```python
from build123d import *

# Parameters (mm, degrees)
SKETCH1_W           = 86
SKETCH1_H           = 40
BOSS_EXTRUDE1_DEPTH = 1.3
SKETCH2_W           = 1.4
SKETCH2_H           = 22
BOSS_EXTRUDE2_DEPTH = 1.3
CUT_EXTRUDE1_DEPTH  = 49.713961038
BOSS_EXTRUDE3_DEPTH = 1.3


with BuildPart() as part:
    # Sketch1 → Boss-Extrude1 (new body)
    with BuildSketch(Plane(origin=(0, 0, 0), x_dir=(1, 0, 0), z_dir=(0, 1, 0))):
        Rectangle(SKETCH1_W, SKETCH1_H)
    extrude(amount=BOSS_EXTRUDE1_DEPTH)

    # Sketch2 → Boss-Extrude2 (add)
    with BuildSketch(Plane(origin=(0, 1.3, 0), x_dir=(1, 0, 0), z_dir=(0, 1, 0))):
        with Locations((-43.7, -3)):
            Rectangle(SKETCH2_W, SKETCH2_H)
        with Locations((43.7, -3)):
            Rectangle(SKETCH2_W, SKETCH2_H)
    extrude(amount=-BOSS_EXTRUDE2_DEPTH)

    # Sketch3 → Cut-Extrude1 (cut, through all)
    with BuildSketch(Plane(origin=(0, 1.3, 0), x_dir=(1, 0, 0), z_dir=(0, 1, 0))):
        Polygon((29, 20), (-29, 20), (-11, -18), (11, -18), align=None)
    extrude(amount=-CUT_EXTRUDE1_DEPTH, mode=Mode.SUBTRACT)

    # Sketch4 → Boss-Extrude3 (add)
    with BuildSketch(Plane(origin=(0, 0, 0), x_dir=(1, 0, 0), z_dir=(0, 1, 0))):
        Polygon((-28, -20), (-18.75, -39.527777778), (18.75, -39.527777778), (28, -20), align=None)
    extrude(amount=BOSS_EXTRUDE3_DEPTH)


solid = part.part
```
Geometry: final body of the model. Coordinates: model frame, mm. A direction names the side the tool comes from. Coordinates: 2 decimals unless noted, no trailing zeros. Order: outer loops, then holes, each group sorted by start corner. A loop starts at its lowest first (then second) coordinate and runs counter-clockwise, first axis right, second up. Notation, with made-up numbers: (59, -34.5) - (101, -34.5) arc R24 ccw to (101, 4.5) - close; hole circle Ø10 at (11.25, 46). An arc over 180 degrees is marked (long way). Write each question's results on one line, items separated by ' | '.
1) Section D-D, the plane z = 29.5. Return loops of the section in (x, y).
Results list:
outline: (-23.5, 0) - (23.5, 0) - (23.5, 1.3) - (-23.5, 1.3) - close
2) Set-up query: faces 1 (the flat face through (-20, 1, -1)), 2 (the flat face through (-1, 0, 23)). Return all of +Z, -Z, +X, -X, +Y, -Y with unobstructed straight access to the full face (end or side cutting, diameter ignored); none if empty.
Results list:
face 1: -Z, +Y, -Y | face 2: +Z, -Z, +X, -X, -Y
3) Line query: line 1 (X direction, y = 0.25, z = -1); line 2 (Z direction, x = 37, y = 0.25); line 3 (Z direction, x = 1, y = 0.95). Output: solid intervals per line, ascending. Write a range as from..to.
Results list:
line 1: -44.4..-20, 20..44.4 | line 2: -20..20 | line 3: 18..39.53
4) Pull-direction query (X, two-part tool) for faces 3 (the flat face through (23.31, 0.64, 29.9)), 4 (the flat face through (-23.44, 0.64, 29.63)), 5 (the flat face through (20, 1, -1)), 6 (the flat face through (-1, 1.3, 23)); classes: pulls with the +X half, pulls with the -X half, needs draft (parallel to the pull), parting line crosses it, or undercut.
Results list:
face 3: pulls with the +X half | face 4: pulls with the -X half | face 5: undercut | face 6: needs draft
5) Section C-C, the plane x = -4. Return loops of the section in (y, z).
Results list:
outline: (0, 18) - (1.3, 18) - (1.3, 39.53) - (0, 39.53) - close
6) Section B-B, the plane y = 0.8. Return loops of the section in (x, z).
Results list:
outline: (-44.4, -8) - (-43, -8) - (-43, -20) - (-29, -20) - (-11, 18) - (11, 18) - (29, -20) - (43, -20) - (43, -8) - (44.4, -8) - (44.4, 14) - (43, 14) - (43, 20) - (28, 20) - (18.75, 39.53) - (-18.75, 39.53) - (-28, 20) - (-43, 20) - (-43, 14) - (-44.4, 14) - close
7) Section A-A, the plane z = -4. Return loops of the section in (x, y), plus the area to 3 significant figures.
Results list:
outline: (-44.4, 0) - (-21.42, 0) - (-21.42, 1.3) - (-44.4, 1.3) - close; (21.42, 0) - (44.4, 0) - (44.4, 1.3) - (21.42, 1.3) - close | area: 59.7 mm^2
8) Pin query (flat end, axial travel): pin 1 (0.6 mm diameter, centred on x = 39, y = 1, fed in from +Z); pin 2 (3 mm diameter, centred on x = -29, z = 15.5, fed in from -Y). Return the tip coordinate at first contact, or that it passes through.
Results list:
pin 1: z = 20 | pin 2: y = 0
